Part model, mm, in its own coordinate system. Face numbers are marked on the shaded views. Round coordinates to 2 decimals unless told otherwise and drop trailing zeros. Loops run counter-clockwise (first coordinate to the right, second up) from the corner with the lowest first, then second, coordinate; pieces in that order, holes last. Notation, with made-up numbers: M -28,-20.5 L 13,-20.5 A7 ccw 13,-9.5 Z; hole C 18.5,36.5 d2. An arc over 180 degrees is marked long. Put each result on its own line as item: value. Start each with the question number.
1) Drop flat-ended pins along their axis: pin 1 Ø0.6 at (y, z) = (30, 0.5) entering from +X; pin 2 Ø5 at (x, y) = (3.5, -3.5) entering from +Z; pin 3 Ø0.6 at (x, z) = (10.5, 4.5) entering from +Y. Give the stop position or say it passes through.
2) Slice it at C-C on z = 5. Give the cut face in (x, y), then the cut area to 3 significant figures.
3) Slice it at A-A on y = 20.5. Give the cut face in (x, z).
4) Pull direction X, two halves, no side cores. Call the marked faces 1, 2 and 3: +X half, -X half, draft (parallel to the pull), parting line (faces both ways), or undercut.
5) Slice it at B-B on x = 6. Give the cut face in (y, z).
6) Probe line 1 along Z through (x, y) = (6.75, 3.5); line 2 along X through (y, z) = (-7, 5.25). List the from-to ranges inside material, lowest first.
```python
from build123d import *

# Parameters (mm, degrees)
F1_DEPTH = 1.1176
F2_W     = 36.874799
F2_H     = 6.35
F3_DEPTH = 1.1176


with BuildPart() as f1:
    # F0 (on Top) → F1 (new body)
    with BuildSketch(Plane.XY):
        Polygon((10.248203, 31.731885), (-5.220397, 31.731885), (-5.220397, -15.308915), (10.248203, -15.308915), (10.248203, -10.228915), (10.248203, 26.651885), align=None)
    extrude(amount=F1_DEPTH)

    # F2 (on face) → F3 (join)
    with BuildSketch(Plane.YZ.offset(10.248203)):
        with Locations((8.208485, 3.175)):
            Rectangle(F2_W, F2_H)
    extrude(amount=F3_DEPTH)


solid = f1.part
```
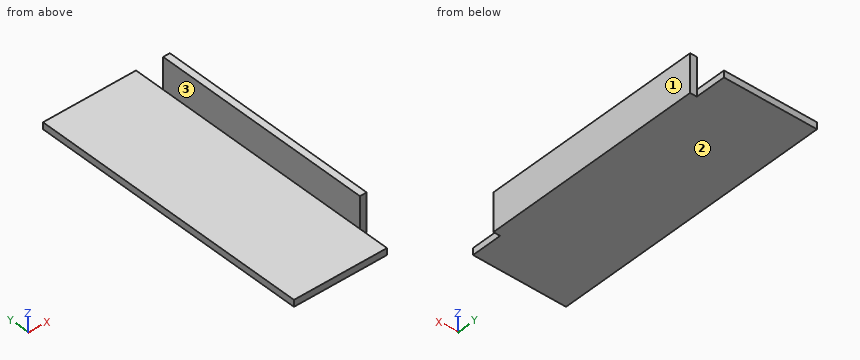
Recorded:
1. pin 1: stops at x = 10.25
1. pin 2: stops at z = 1.12
1. pin 3: stops at y = 26.65
2. outline: M 10.25,-10.23 L 11.37,-10.23 L 11.37,26.65 L 10.25,26.65 Z
2. area: 41.2 mm2
3. outline: M -5.22,0 L 11.37,0 L 11.37,6.35 L 10.25,6.35 L 10.25,1.12 L -5.22,1.12 Z
4. face 1: +X half
4. face 2: draft
4. face 3: -X half
5. outline: M -15.31,0 L 31.73,0 L 31.73,1.12 L -15.31,1.12 Z
6. line 1: z = 0 to 1.12
6. line 2: x = 10.25 to 11.37
